Could you check a few things on this model? Use its own coordinates, in mm. A direction names the side the tool comes from. Round coordinates to 2 decimals unless told otherwise and drop trailing zeros. Loops run counter-clockwise (first coordinate to the right, second up) from the corner with the lowest first, then second, coordinate; pieces in that order, holes last. Notation, with made-up numbers: (35.25, 12.5) - (75.25, 12.5) arc R20 ccw to (75.25, 17.5) - close; hole circle Ø8 at (46.25, 63.25). An arc over 180 degrees is marked (long way). Use one line per item in the form item = value.
Autodesk Inventor part; units mm, degrees
ref_plane "YZ Plane" through (0, 0, 0) normal (1, 0, 0) x (0, 1, 0)
ref_plane "XY Plane" through (0, 0, 0) normal (0, 0, 1) x (1, 0, 0)
sketch "Sketch1" plane through (0, 0, 0) normal (0, 0, 1) x (1, 0, 0)
  line L0 (-67, 3) -> (-67, -3)
  line L1 (-67, -3) -> (-3, -3)
  line L2 (-67, 3) -> (-3, 3)
  line L3 (0, -3) -> (0, 3) construction
  line L4 (3, -3) -> (3, 3)
  line L5 (-3, 3) -> (-3, -3)
  arc A0 (-3, -3) -> (3, -3) centre (0, -3) ccw
  arc A1 (3, 3) -> (-3, 3) centre (0, 3) ccw
  point P0 (0, 0)
  point P1 (-3, -3)
  dimension "d0" = 70
  dimension "d1" = 3
  dimension "d2" = 6
  dimension "d3" = 6
extrude "Extrusion1" add sketch "Sketch1" along normal mid plane 140
sketch "Sketch2" plane through (-67, 3, 70) normal (0, 1, 0) x (1, 0, 0)
  line L0 (0, 0) -> (64, 0)
  line L1 (64, 0) -> (44, 0)
  line L2 (0, 140) -> (0, 0)
  line L3 (44, 0) -> (34, 10)
  line L4 (34, 10) -> (34, 29.9)
  line L5 (34, 29.9) -> (0, 53.7071)
  line L6 (0, 53.7071) -> (0, 86.2929)
  line L7 (0, 86.2929) -> (34, 110.1)
  line L8 (34, 110.1) -> (34, 130)
  line L9 (34, 130) -> (44, 140)
  line L10 (0, 140) -> (64, 140)
  line L11 (44, 140) -> (64, 140)
  line L12 (64, 140) -> (64, 0)
  point P0 (67, 70)
  dimension "d6" = 20
  dimension "d7" = 20
  dimension "d8" = 30
  dimension "d9" = 45
  dimension "d10" = 45
  dimension "d11" = 19.9
  dimension "d12" = 19.9
  dimension "d13" = 125
  dimension "d14" = 125
extrude "Extrusion2" cut sketch "Sketch2" against normal through all contours L2 L5 L4 L3 L0 | L2 L10 L9 L8 L7
sketch "Sketch3" plane through (-3, 3, 70) normal (0, 1, 0) x (1, 0, 0)
  circle A0 centre (-59, 80) radius 1.9
  circle A1 centre (-59, 60) radius 1.9
  line L0 (-64, 86.2929) -> (-64, 53.7071)
  line L1 (-59, 80) -> (-59, 60)
  point P0 (3, 70)
  point P1 (-64, 70)
  dimension "d17" = 3.8
  dimension "d18" = 3.8
  dimension "d19" = 20
  dimension "d20" = 10
  dimension "d21" = 5
extrude "Extrusion3" cut sketch "Sketch3" against normal through all
sketch "Sketch4" plane through (-3, 3, 70) normal (0, 1, 0) x (1, 0, 0)
  line L0 (-44.67, 64.05) -> (-12.45, 64.05)
  line L1 (-12.45, 64.05) -> (-12.45, 75.95)
  line L2 (-12.45, 75.95) -> (-44.67, 75.95)
  line L3 (-44.67, 75.95) -> (-44.67, 64.05)
  line L4 (-44.67, 64.05) -> (-12.45, 75.95) construction
  line L5 (-12.45, 64.05) -> (-44.67, 75.95) construction
  line L6 (6, 140) -> (6, 0)
  line L7 (6, 70) -> (-4, 70)
  line L8 (-40.17, 64.05) -> (-16.95, 64.05)
  line L9 (-16.95, 64.05) -> (-16.95, 75.95)
  line L10 (-16.95, 75.95) -> (-40.17, 75.95)
  line L11 (-40.17, 75.95) -> (-40.17, 64.05)
  line L12 (0, 140) -> (0, 0)
  line L13 (-44.87, 76.15) -> (-12.25, 76.15)
  line L14 (-12.25, 76.15) -> (-12.25, 63.85)
  line L15 (-12.25, 63.85) -> (-44.87, 63.85)
  line L16 (-44.87, 63.85) -> (-44.87, 76.15)
  line L17 (-47.37, 78.65) -> (-47.37, 61.35)
  line L18 (-9.75, 61.35) -> (-9.75, 78.65)
  circle A0 centre (-59, 80) radius 1.9
  circle A1 centre (-59, 60) radius 1.9
  line L19 (-47.37, 61.35) -> (-60.337, 61.35)
  line L20 (-57.663, 61.35) -> (-9.75, 61.35)
  line L21 (-9.75, 78.65) -> (-57.663, 78.65)
  line L22 (-60.337, 78.65) -> (-47.37, 78.65)
  circle A2 centre (-29, 70) radius 2.45
  point P0 (3, 70)
  point P1 (-28.56, 70)
  point P2 (-47.37, 78.65)
  point P3 (-47.37, 61.35)
  point P4 (-57.663, 61.35)
  point P5 (-57.663, 78.65)
  dimension "d24" = 32.22
  dimension "d25" = 11.9
  dimension "d26" = 4.5
  dimension "d27" = 4.5
  dimension "d30" = 0.2
  dimension "d34" = 2.5
  dimension "d35" = 2.5
  dimension "d36" = 2.5
  dimension "d37" = 2.5
  dimension "d51" = 29
  dimension "d52" = 12.05
  dimension "d53" = 4.9
extrude "Extrusion4" add sketch "Sketch4" against normal blind 15 contours L3 L2 L11 L0 | L11 L2 L9 L0 | L9 L2 L1 L0 | L13 L14 L15 L16 | L21 L18 L20 L17 | A2
sketch "Sketch5" plane through (-3, -12, 70) normal (0, -1, 0) x (1, 0, 0)
  circle A0 centre (-59, -80) radius 1.9
  circle A1 centre (-59, -60) radius 1.9
  line L0 (-30, -110.1) -> (-64, -86.2929)
  line L1 (-64, -86.2929) -> (-64, -53.7071)
  line L2 (-64, -53.7071) -> (-30, -29.9)
  line L3 (-30, -29.9) -> (-30, -10)
  line L4 (-30, -10) -> (-20, 0)
  line L5 (0, 0) -> (-20, 0)
  line L6 (0, -140) -> (0, 0)
  line L7 (-20, -140) -> (0, -140)
  line L8 (-20, -140) -> (-30, -130)
  line L9 (-30, -130) -> (-30, -110.1)
  line L10 (-12.45, -75.95) -> (-44.67, -75.95)
  line L11 (-16.95, -64.05) -> (-16.95, -75.95)
  line L12 (-44.87, -76.15) -> (-12.25, -76.15)
  line L13 (-12.25, -76.15) -> (-12.25, -63.85)
  line L14 (-12.45, -64.05) -> (-12.45, -75.95)
  line L15 (-44.67, -64.05) -> (-12.45, -64.05)
  line L16 (-12.25, -63.85) -> (-44.87, -63.85)
  line L17 (-44.87, -63.85) -> (-44.87, -76.15)
  line L18 (-44.67, -75.95) -> (-44.67, -64.05)
  line L19 (-44.67, -64.05) -> (-12.45, -75.95) construction
  line L20 (-40.17, -75.95) -> (-40.17, -64.05)
  line L21 (-40.17, -75.95) -> (-40.17, -76.15)
  line L22 (-40.17, -64.05) -> (-40.17, -63.85)
  line L23 (-16.95, -76.15) -> (-16.95, -75.95)
  line L24 (-16.95, -64.05) -> (-16.95, -63.85)
  point P0 (3, -70)
extrude "Extrusion5" cut sketch "Sketch5" against normal blind 7 contours L14 L15 L24 L16 L13 L12 L23 L10 | L10 L11 L15 L14 | L23 L12 L21 L10 | L10 L20 L15 L11 | L21 L12 L17 L16 L22 L15 L18 L10 | L10 L18 L15 L20 | L15 L22 L16 L24
sketch "Sketch6" plane through (-3, -5, 70) normal (0, -1, 0) x (1, 0, 0)
  line L0 (-16.95, -64.05) -> (-16.95, -75.95) construction
  line L1 (-12.45, -64.05) -> (-44.67, -75.95) construction
  line L2 (-40.17, -75.95) -> (-40.17, -64.05) construction
  line L3 (-12.25, -63.85) -> (-12.25, -76.15)
  line L4 (-44.87, -63.85) -> (-12.25, -63.85)
  line L5 (-44.87, -76.15) -> (-44.87, -63.85)
  line L6 (-12.25, -76.15) -> (-44.87, -76.15)
  line L7 (-16.95, -64.05) -> (-16.95, -63.85)
  line L8 (-44.87, -63.85) -> (-12.25, -63.85)
  line L9 (-16.95, -75.95) -> (-16.95, -76.15)
  line L10 (-40.17, -76.15) -> (-40.17, -75.95)
  line L11 (-40.17, -64.05) -> (-40.17, -63.85)
  line L12 (-40.32, -76.15) -> (-40.32, -63.85)
  line L13 (-16.8, -76.15) -> (-16.8, -63.85)
  line L14 (-40.32, -76.15) -> (-16.8, -76.15)
  line L15 (-16.8, -76.15) -> (-16.8, -63.85)
  line L16 (-16.8, -63.85) -> (-40.32, -63.85)
  line L17 (-40.32, -63.85) -> (-40.32, -76.15)
  point P0 (3, -70)
  dimension "d40" = 0.15
  dimension "d41" = 0.15
extrude "Extrusion6" cut sketch "Sketch6" against normal blind 5 contours L13 L6 L12 L4
sketch "Sketch7" plane through (-3, 0, 70) normal (0, -1, 0) x (1, 0, 0)
  line L0 (-16.8, -63.85) -> (-16.8, -76.15)
  line L1 (-16.8, -70) -> (-21, -70)
  circle A0 centre (-22.95, -70) radius 6.15 construction
  line L2 (-44.87, -63.85) -> (-12.25, -63.85)
  arc A1 (-24.3166, -63.85) -> (-24.3166, -76.15) centre (-22.95, -70) ccw
  circle A2 centre (-28.8, -70) radius 3 construction
  line L3 (-24.3166, -63.85) -> (-30.3313, -67.4202) construction
  line L4 (-30.3313, -72.5798) -> (-24.3166, -76.15) construction
  line L5 (-12.25, -76.15) -> (-44.87, -76.15)
  arc A3 (-21.5834, -63.85) -> (-24.3166, -63.85) centre (-22.95, -70) ccw construction
  arc A4 (-21.5834, -76.15) -> (-16.8, -71.3666) centre (-22.95, -70) ccw
  arc A5 (-24.3166, -76.15) -> (-21.5834, -76.15) centre (-22.95, -70) ccw construction
  arc A6 (-16.8, -71.3666) -> (-16.8, -68.6334) centre (-22.95, -70) ccw construction
  arc A7 (-16.8, -68.6334) -> (-21.5834, -63.85) centre (-22.95, -70) ccw
  line L6 (-26.1657, -64.5825) -> (-30.4916, -67.1503)
  arc A8 (-28.169, -66.7467) -> (-28.3286, -66.7197) centre (-28.8, -70) ccw
  arc A9 (-30.4916, -67.1503) -> (-30.4916, -72.8497) centre (-28.8, -70) ccw
  line L7 (-30.4916, -72.8497) -> (-26.1657, -75.4175)
  point P0 (3, -70)
  dimension "d44" = 0.15
  dimension "d45" = 6
  dimension "d46" = 12
extrude "Extrusion7" cut sketch "Sketch7" against normal through all contours L0 A4 L5 A1 L2 A7 | A1 L7 A9 L6
fillet "Fillet1" radius 2 4 edges at (-12.75, -7.5, -8.65) (-50.37, -7.5, -8.65) (-50.37, -7.5, 8.65) (-12.75, -7.5, 8.65)
sketch "Sketch9" plane through (-3, -5, 70) normal (0, -1, 0) x (1, 0, 0)
  circle A0 centre (-14.81, -70) radius 0.8
  line L0 (3, -70) -> (-41.3866, -70) construction
  line L1 (-40.32, -76.15) -> (-40.32, -63.85)
  line L2 (6, -140) -> (6, 0)
  circle A1 centre (-42.31, -70) radius 0.8
  dimension "d64" = 1.6
  dimension "d65" = 20.81
  dimension "d66" = 1.6
  dimension "d67" = 27.5
extrude "Extrusion9" cut sketch "Sketch9" against normal blind 6
sketch "Sketch10" plane through (-3, -5, 70) normal (0, -1, 0) x (1, 0, 0)
  circle A0 centre (-14.81, -70) radius 0.8
  circle A1 centre (-42.31, -70) radius 0.8
  line L0 (-12.4678, -70) -> (-46, -70)
  line L1 (-44.87, -63.85) -> (-12.25, -63.85)
  line L2 (-12.25, -63.85) -> (-12.25, -76.15)
  line L3 (-12.25, -76.15) -> (-44.87, -76.15)
  line L4 (-44.87, -76.15) -> (-44.87, -63.85)
  arc A2 (-9.75, -63.35) -> (-11.75, -61.35) centre (-11.75, -63.35) ccw
  line L5 (-11.75, -61.35) -> (-45.37, -61.35)
  arc A3 (-45.37, -61.35) -> (-47.37, -63.35) centre (-45.37, -63.35) ccw
  line L6 (-47.37, -63.35) -> (-47.37, -76.65)
  arc A4 (-47.37, -76.65) -> (-45.37, -78.65) centre (-45.37, -76.65) ccw
  line L7 (-45.37, -78.65) -> (-11.75, -78.65)
  arc A5 (-11.75, -78.65) -> (-9.75, -76.65) centre (-11.75, -76.65) ccw
  line L8 (-9.75, -76.65) -> (-9.75, -63.35)
  line L9 (-10.75, -63.35) -> (-10.75, -76.65)
  line L10 (-46.37, -64) -> (-46.37, -74.4084)
  circle A6 centre (-43.87, -70) radius 2.5
  circle A7 centre (-13.25, -70) radius 2.5
  point P0 (3, -70)
  point P1 (-44.87, -67.7087)
  point P2 (-44.87, -72.2913)
  point P3 (-12.25, -67.7087)
  point P4 (-12.25, -72.2913)
  dimension "d70" = 1
  dimension "d71" = 1
  dimension "d72" = 5
  dimension "d73" = 5
extrude "Extrusion10" cut sketch "Sketch10" along normal through all contours A7 L2 | L4 A6 picked at (-11.5834, -70.097)
chamfer "Chamfer1" distance 1 angle 45 4 edges at (-15.25, -8.5, 2.2913) (-15.25, -8.5, -2.2913) (-47.87, -8.5, -2.2913) (-47.87, -8.5, 2.2913)
equation "\"d7\" = d6"
equation "\"d10\" = d9"
equation "\"d12\" = d11"
equation "\"d14\" = d13"
equation "\"d17\" = d18"
equation "\"d27\" = d26"
equation "\"d34\" = d36"
equation "\"d35\" = d36"
equation "\"d37\" = d36"
properties part number "gripper_head 1"
1. Please list where these lines run through material, in increasing order: line 1 along Z through (x, y) = (-62, -1.2); line 2 along Y through (x, z) = (-44.5, 0.5); line 3 along Z through (x, y) = (-26.5, -9.75).
Solution:
line_1 = -19.79 to -11.9, -8.1 to 8.1, 11.9 to 19.79
line_2 = -5 to 3
line_3 = -8.65 to -6.15, 6.15 to 8.65
2. If we section it at A-A, the plane z = 10: Write out the boundary of the cut face in (x, y).
Solution:
outline = (-67, -3) - (-63.9, -3) - (-63.9, 3) - (-67, 3) - close; (-60.1, -3) - (-3, -3) arc R3 ccw to (3, -3) - (3, 3) arc R3 ccw to (-3, 3) - (-60.1, 3) - close
3. If we section it at D-D, the plane y = 4.5: Write out the boundary of the cut face in (x, z), plus the area to 3 significant figures.
Solution:
outline = (-2.6, -70) - (2.6, -70) - (2.6, 70) - (-2.6, 70) - close
area = 727 mm^2
4. If we section it at B-B, the plane z = -46: Write out the boundary of the cut face in (x, y), plus the area to 3 significant figures.
Solution:
outline = (-33, -3) - (-3, -3) arc R3 ccw to (3, -3) - (3, 3) arc R3 ccw to (-3, 3) - (-33, 3) - close
area = 244 mm^2
5. If we section it at C-C, the plane x = 0: Write out the boundary of the cut face in (y, z).
Solution:
outline = (-6, -70) - (6, -70) - (6, 70) - (-6, 70) - close
6. For P1, Ø7, axis at y = -9, z = 3, coming from the +X side; P2, Ø1.3, axis at x = -17.5, z = -0.5, coming from the -Y side; P3, Ø1.4, axis at y = -9.5, z = -4.5, coming from the +X side; P4, Ø4, axis at x = -23.5, z = 3, coming from the -Y side, each with a flat end and sliding along its axis, tell me the tip position at first contact or that it passes through.
Solution:
P1 = 1.66
P2 = -5
P3 = -12.75
P4 = through
7. On a 3-axis mill with a long thin cutter (end or side, diameter ignored), from which of +Z, -Z, +X, -X, +Y, -Y can I reach the whole of each face in a straight line? I mean faces 4 (the face through (-35.4, 3, -1)), 5 (the face through (-31, -7, -8.65)), 6 (the face through (-13.75, -8.45, 0.03)). Say none if no direction works.
Solution:
face_4 = +Z, -Z, -X, +Y
face_5 = -Z, -X, -Y
face_6 = -Y
8. We'd pull the mould along Z, two halves only. Please class faces 1 (the face through (-32, -7, 8.65)), 2 (the face through (-37, 0, 0)), 3 (the face through (-12.75, -7, 0)): +Z half, -Z half, draft (parallel to the pull), parting line (faces both ways), or undercut.
Solution:
face_1 = +Z half
face_2 = undercut
face_3 = draft
